from build123d import *

# Parameters (mm, degrees)
SKETCH1_W               = 30
SKETCH1_H               = 30
BOSS_EXTRUDE1_DEPTH     = 1
SKETCH2_R               = 12.4
CUT_EXTRUDE1_DEPTH      = 22.236760582
SKETCH4_W               = 2
SKETCH4_H               = 4
SKETCH4_W_2             = 4
SKETCH4_H_2             = 2
BOSS_EXTRUDE2_DEPTH     = 2
SKETCH5_W               = 4
SKETCH5_H               = 0.5
BOSS_EXTRUDE3_DEPTH     = 0.8
SKETCH6_W               = 4
SKETCH6_H               = 0.5
BOSS_EXTRUDE4_DEPTH     = 0.8
SKETCH7_W               = 4
SKETCH7_H               = 0.5
BOSS_EXTRUDE5_DEPTH     = 0.8
SKETCH8_W               = 4
SKETCH8_H               = 0.5
BOSS_EXTRUDE6_DEPTH     = 0.8
SKETCH11_W              = 38.930666634
SKETCH11_H              = 2
BOSS_EXTRUDE9_DEPTH     = 10
BOSS_EXTRUDE10_DEPTH    = 30
BOSS_EXTRUDE11_DEPTH    = 30
CUT_EXTRUDE2_DEPTH      = 45.684189659
CUT_EXTRUDE2_DEPTH_BACK = 45.684189659
SKETCH14_W              = 8.930666634
SKETCH14_H              = 10
SKETCH15_W              = 29.996322287
SKETCH15_H              = 1
BOSS_EXTRUDE12_DEPTH    = 5
SKETCH20_W              = 30
SKETCH20_H              = 3.6732435
BOSS_EXTRUDE16_DEPTH    = 90
CUT_EXTRUDE3_DEPTH      = 80.886258607
SKETCH23_W              = 30
SKETCH23_H              = 55.569719249
CUT_EXTRUDE5_DEPTH      = 10
SKETCH24_W              = 30
SKETCH24_H              = 3.6732435
BOSS_EXTRUDE17_DEPTH    = 76.2
SKETCH25_W              = 30
SKETCH25_H              = 3.6732435
CUT_EXTRUDE6_DEPTH      = 25.4
SKETCH26_W              = 30
SKETCH26_H              = 3.6732435
BOSS_EXTRUDE18_DEPTH    = 17.8
SKETCH27_W              = 30
SKETCH27_H              = 71.821297676
CUT_EXTRUDE7_DEPTH      = 10
SKETCH28_R              = 3.375
CUT_EXTRUDE8_DEPTH      = 10


with BuildPart() as part:
    # Sketch1 → Boss-Extrude1 (new body)
    with BuildSketch(Plane(origin=(0, 0, 0), x_dir=(1, 0, 0), z_dir=(0, 1, 0))):
        Rectangle(SKETCH1_W, SKETCH1_H)
    extrude(amount=BOSS_EXTRUDE1_DEPTH)

    # Sketch2 → Cut-Extrude1 (cut, through all)
    with BuildSketch(Plane(origin=(0, 1, 0), x_dir=(1, 0, 0), z_dir=(0, 1, 0))):
        with Locations(Location((0, 0, 0), (0, 0, 270))):
            Circle(SKETCH2_R)
    extrude(amount=-CUT_EXTRUDE1_DEPTH, mode=Mode.SUBTRACT)

    # Sketch4 → Boss-Extrude2 (add)
    with BuildSketch(Plane(origin=(0, 1, 0), x_dir=(1, 0, 0), z_dir=(0, 1, 0))):
        with Locations((13.7, 0)):
            Rectangle(SKETCH4_W, SKETCH4_H)
        with Locations((-13.7, 0)):
            Rectangle(SKETCH4_W, SKETCH4_H)
        with Locations((0, 13.7)):
            Rectangle(SKETCH4_W_2, SKETCH4_H_2)
        with Locations((0, -13.7)):
            Rectangle(SKETCH4_W_2, SKETCH4_H_2)
    extrude(amount=BOSS_EXTRUDE2_DEPTH)

    # Sketch5 → Boss-Extrude3 (add)
    with BuildSketch(Plane.ZY.offset(-12.7)):
        with Locations((0, 2.75)):
            Rectangle(SKETCH5_W, SKETCH5_H)
    extrude(amount=BOSS_EXTRUDE3_DEPTH)

    # Sketch6 → Boss-Extrude4 (add)
    with BuildSketch(Plane(origin=(0, 0, 12.7), x_dir=(-1, 0, 0), z_dir=(0, 0, -1))):
        with Locations((0, 2.75)):
            Rectangle(SKETCH6_W, SKETCH6_H)
    extrude(amount=BOSS_EXTRUDE4_DEPTH)

    # Sketch7 → Boss-Extrude5 (add)
    with BuildSketch(Plane(origin=(-12.7, 0, 0), x_dir=(0, 0, -1), z_dir=(1, 0, 0))):
        with Locations((0, 2.75)):
            Rectangle(SKETCH7_W, SKETCH7_H)
    extrude(amount=BOSS_EXTRUDE5_DEPTH)

    # Sketch8 → Boss-Extrude6 (add)
    with BuildSketch(Plane.XY.offset(-12.7)):
        with Locations((0, 2.75)):
            Rectangle(SKETCH8_W, SKETCH8_H)
    extrude(amount=BOSS_EXTRUDE6_DEPTH)

    # Sketch11 → Boss-Extrude9 (add)
    with BuildSketch(Plane.XZ):
        with Locations((4.465333317, -16)):
            Rectangle(SKETCH11_W, SKETCH11_H)
    extrude(amount=-BOSS_EXTRUDE9_DEPTH)



with BuildPart() as body_2:
    # Sketch12 → Boss-Extrude10 (new body)
    with BuildSketch(Plane.ZY.offset(15)):
        Polygon((-17, 10), (-25.602361573, -20), (-30.365256607, -18.634261826), (-21.762895034, 11.365738174), align=None)
    extrude(amount=-BOSS_EXTRUDE10_DEPTH)


with BuildPart() as part_1:
    add(part.part)

    add(body_2.part)  # Boss-Extrude11 merges body 2
    # Sketch13 → Boss-Extrude11 (add)
    with BuildSketch(Plane.ZY.offset(15)):
        Polygon((-17, 0), (-25.021968012, 0), (-21.762895034, 11.365738174), (-17, 10), align=None)
    extrude(amount=-BOSS_EXTRUDE11_DEPTH)

    # Sketch14 → Cut-Extrude2 (cut, two sides: drawn at the far end of the back side and taken through both)
    with BuildSketch(Plane(origin=(0, 0, -17), x_dir=(-1, 0, 0), z_dir=(0, 0, -1)).offset(-CUT_EXTRUDE2_DEPTH_BACK)):
        with Locations((-19.465333317, 5)):
            Rectangle(SKETCH14_W, SKETCH14_H)
    extrude(amount=CUT_EXTRUDE2_DEPTH + CUT_EXTRUDE2_DEPTH_BACK, mode=Mode.SUBTRACT)

    # Sketch15 → Boss-Extrude12 (add)
    with BuildSketch(Plane.XY.offset(15)):
        with Locations((0.001838857, 0.5)):
            Rectangle(SKETCH15_W, SKETCH15_H)
    extrude(amount=BOSS_EXTRUDE12_DEPTH)

    # Sketch20 → Boss-Extrude16 (add)
    with BuildSketch(Plane(origin=(0, -25.264073265, -7.244356434), x_dir=(1, 0, 0), z_dir=(0, -0.9612616959383165, -0.2756373558170081))):
        with Locations((0, -20.934444139)):
            Rectangle(SKETCH20_W, SKETCH20_H)
    extrude(amount=-BOSS_EXTRUDE16_DEPTH)

    # Sketch21 → Cut-Extrude3 (cut, through all)
    with BuildSketch(Plane(origin=(15, 0, 0), x_dir=(0, 0, -1), z_dir=(1, 0, 0))):
        Polygon((21.762895034, 11.365738174), (20.530948276, 11.012483126), (29.133309849, -18.987516874), (30.365256607, -18.634261826), align=None)
    extrude(amount=-CUT_EXTRUDE3_DEPTH, mode=Mode.SUBTRACT)

    # Sketch23 → Cut-Extrude5 (cut)
    with BuildSketch(Plane(origin=(0, 6.276556391, -21.888953415), x_dir=(-1, 0, 0), z_dir=(0, 0.2756373558170081, -0.9612616959383165))):
        with Locations((0, 35.932939211)):
            Rectangle(SKETCH23_W, SKETCH23_H)
    extrude(amount=-CUT_EXTRUDE5_DEPTH, mode=Mode.SUBTRACT)

    # Sketch24 → Boss-Extrude17 (add)
    with BuildSketch(Plane(origin=(0, 7.832436802, 2.245915112), x_dir=(1, 0, 0), z_dir=(0, 0.9612616959383165, 0.2756373558170081))):
        with Locations((0, 20.934444139)):
            Rectangle(SKETCH24_W, SKETCH24_H)
    extrude(amount=BOSS_EXTRUDE17_DEPTH)

    # Sketch25 → Cut-Extrude6 (cut)
    with BuildSketch(Plane(origin=(0, 81.080578032, 23.249481625), x_dir=(1, 0, 0), z_dir=(0, 0.9612616959383165, 0.27563735581700777))):
        with Locations((0, 20.934444139)):
            Rectangle(SKETCH25_W, SKETCH25_H)
    extrude(amount=-CUT_EXTRUDE6_DEPTH, mode=Mode.SUBTRACT)

    # Sketch26 → Boss-Extrude18 (add)
    with BuildSketch(Plane(origin=(0, 56.664530955, 16.248292788), x_dir=(1, 0, 0), z_dir=(0, 0.9612616959383156, 0.2756373558170107))):
        with Locations((0, 20.934444139)):
            Rectangle(SKETCH26_W, SKETCH26_H)
    extrude(amount=BOSS_EXTRUDE18_DEPTH)

    # Sketch27 → Cut-Extrude7 (cut)
    with BuildSketch(Plane(origin=(0, 5.264073265, -18.358005138), x_dir=(1, 0, 0), z_dir=(0, -0.2756373558170081, 0.9612616959383165))):
        with Locations((0, 40.837430748)):
            Rectangle(SKETCH27_W, SKETCH27_H)
    extrude(amount=-CUT_EXTRUDE7_DEPTH, mode=Mode.SUBTRACT)

    # Sketch28 → Cut-Extrude8 (cut)
    with BuildSketch(Plane(origin=(0, 5.264073265, -18.358005138), x_dir=(1, 0, 0), z_dir=(0, -0.27563735581700294, 0.9612616959383178))):
        with Locations(Location((0, -19.05, 0), (0, 0, 270))):
            Circle(SKETCH28_R)
    extrude(amount=-CUT_EXTRUDE8_DEPTH, mode=Mode.SUBTRACT)


solid = part_1.part
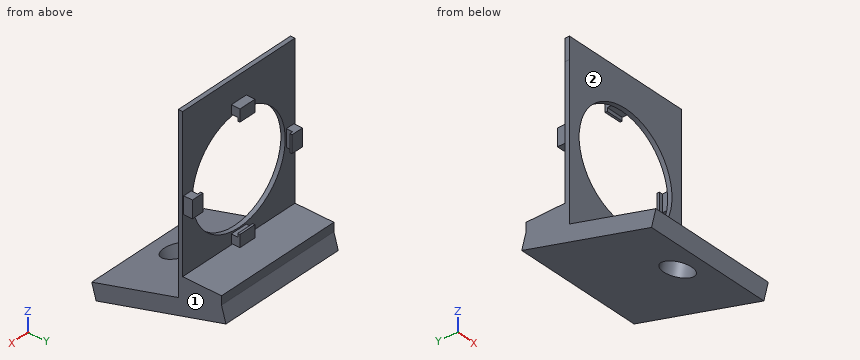
Verification items for the finished model (mm, model axes). Face numbers are marked on the shaded views. A direction names the side the tool comes from. Round coordinates to 2 decimals unless told otherwise and drop trailing zeros. Write each loop counter-clockwise with the first axis right and the second up, starting at its lowest first coordinate (ties: lowest second). Pieces come first, ordered by that corner, then holes.
(1) Section check A-A (z = 0). Enter the section's corners in (x, y).
Returned:
outline: (-15, 0) - (-12.4, 0) - (-12.4, 1) - (-12.7, 1) - (-12.7, 2.5) - (-11.9, 2.5) - (-11.9, 3) - (-14.7, 3) - (-14.7, 1) - (-15, 1) - close; (11.9, 2.5) - (12.7, 2.5) - (12.7, 1) - (12.4, 1) - (12.4, 0) - (15, 0) - (15, 1) - (14.7, 1) - (14.7, 3) - (11.9, 3) - close
(2) Depth check by flat-ended pin: pin 1 Ø0.5 at (y, z) = (0.5, 18.5) entering from -X; pin 2 Ø0.9 at (x, z) = (12, -0.5) entering from -Y; pin 3 Ø5 at (x, y) = (10, 4) entering from -Z; pin 4 Ø7 at (x, y) = (-7, 4) entering from +Z. Enter the tip coordinate at first touch or a pass-through.
Returned:
pin 1: stops at x = -15
pin 2: stops at y = 0
pin 3: stops at z = -23.26
pin 4: stops at z = 20
(3) Material ranges on line 1 (X direction, y = 0.3, z = 0); line 2 (Y direction, x = 13, z = -13); line 3 (Y direction, x = 0, z = -14), recorded low to high.
Returned:
line 1: x = -15 to -12.4, 12.4 to 15
line 2: y = 0 to 1
line 3: y = 0 to 3
(4) Section check C-C (x = -5.5). Enter the section's corners in (y, z), plus the area to 3 significant figures.
Returned:
outline: (-20, -25.6) - (-18.99, -29.13) - (11.01, -20.53) - (10, -17) - (10, -15) - (1, -15) - (1, -11.11) - (0, -11.11) - (0, -19.87) - close; (0, 11.11) - (1, 11.11) - (1, 20) - (0, 20) - close
area: 162 mm2
(5) Section check D-D (z = -7). Enter the section's corners in (x, y).
Returned:
outline: (-15, 0) - (-10.24, 0) - (-10.24, 1) - (-15, 1) - close; (10.24, 0) - (15, 0) - (15, 1) - (10.24, 1) - close
(6) Section check B-B (x = 0). Give the number of separate pieces and of enclosed holes in the cut face, plus the area to 3 significant figures.
Returned:
separate pieces: 3
enclosed holes: 0
area: 143 mm2
(7) Access from +Z, -Z, +X, -X, +Y, -Y to the whole of each face (thin tool, end or side, straight path). Record for the marked faces 1 and 2.
Returned:
face 1: +Z, -Z, +X, +Y, -Y
face 2: +Z, +X, -X, -Y
